Design review of the part built by this model. Coordinates are the model's own, in mm. A direction names the side the tool comes from. Round coordinates to 2 decimals unless told otherwise and drop trailing zeros. Loops run counter-clockwise (first coordinate to the right, second up) from the corner with the lowest first, then second, coordinate; pieces in that order, holes last. Notation, with made-up numbers: M -22,72.25 L 24,72.25 A29 ccw 24,105.25 Z; hole C 87,81 d6. An arc over 180 degrees is marked long. Answer as CSV lines item,"result". Start each with the question number.
Autodesk Inventor part; units mm, degrees
ref_plane "YZ Plane" through (0, 0, 0) normal (1, 0, 0) x (0, 1, 0)
ref_plane "XZ Plane" through (0, 0, 0) normal (0, 1, 0) x (-1, 0, 0)
ref_plane "XY Plane" through (0, 0, 0) normal (0, 0, 1) x (1, 0, 0)
sketch "Sketch1" plane through (0, 0, 0) normal (0, 1, 0) x (-1, 0, 0)
  line L0 (45.72, 0) -> (45.72, -69.85)
  line L1 (0, -69.85) -> (0, 0)
  line L2 (45.72, -69.85) -> (58.42, -69.85)
  line L3 (58.42, -69.85) -> (58.42, -82.55)
  line L4 (58.42, -82.55) -> (45.72, -82.55)
  line L5 (45.72, -82.55) -> (45.72, -69.85)
  line L6 (45.72, 0) -> (58.42, 0)
  line L7 (58.42, 0) -> (58.42, 12.7)
  line L8 (58.42, 12.7) -> (45.72, 12.7)
  line L9 (45.72, 12.7) -> (45.72, 0)
  line L10 (0, 0) -> (-12.7, 0)
  line L11 (-12.7, 0) -> (-12.7, 12.7)
  line L12 (-12.7, 12.7) -> (0, 12.7)
  line L13 (0, 12.7) -> (0, 0)
  line L14 (0, -69.85) -> (-12.7, -69.85)
  line L15 (-12.7, -69.85) -> (-12.7, -82.55)
  line L16 (-12.7, -82.55) -> (0, -82.55)
  line L17 (0, -82.55) -> (0, -69.85)
  line L18 (0, 0) -> (0, 6.35)
  line L19 (0, 6.35) -> (45.72, 6.35)
  line L20 (45.72, 6.35) -> (45.72, 0)
  line L21 (0, -69.85) -> (0, -76.2)
  line L22 (0, -76.2) -> (45.72, -76.2)
  line L23 (45.72, -76.2) -> (45.72, -69.85)
  line L24 (45.72, -69.85) -> (52.07, -69.85)
  line L25 (52.07, -69.85) -> (52.07, 0)
  line L26 (52.07, 0) -> (45.72, 0)
  line L27 (45.72, 0) -> (45.72, -69.85)
  line L28 (0, 0) -> (-8.636, 0)
  line L29 (-8.636, 0) -> (-8.636, -69.85)
  line L30 (-8.636, -69.85) -> (0, -69.85)
  line L31 (0, -69.85) -> (0, 0)
  line L32 (0, 3.175) -> (0, -9.525)
  line L33 (45.72, -9.525) -> (45.72, 3.175)
  line L34 (0, -73.025) -> (0, -60.325)
  line L35 (45.72, -60.325) -> (45.72, -73.025)
  line L36 (34.29, -60.325) -> (11.43, -60.325)
  line L37 (11.43, -60.325) -> (11.43, -73.025)
  line L38 (11.43, -73.025) -> (34.29, -73.025)
  line L39 (34.29, -73.025) -> (34.29, -60.325)
  line L40 (34.29, -9.525) -> (11.43, -9.525)
  line L41 (11.43, -9.525) -> (11.43, 3.175)
  line L42 (11.43, 3.175) -> (34.29, 3.175)
  line L43 (34.29, 3.175) -> (34.29, -9.525)
  line L44 (11.43, -3.175) -> (7.62, -3.175)
  line L45 (7.62, -3.175) -> (7.62, -6.985)
  line L46 (7.62, -6.985) -> (11.43, -6.985)
  line L47 (11.43, -6.985) -> (11.43, -3.175)
  line L48 (0, -6.985) -> (3.81, -6.985)
  line L49 (3.81, -6.985) -> (3.81, -10.795)
  line L50 (3.81, -10.795) -> (0, -10.795)
  line L51 (0, -10.795) -> (0, -6.985)
  line L52 (38.1, -62.865) -> (34.29, -62.865)
  line L53 (38.1, -66.675) -> (38.1, -62.865)
  line L54 (34.29, -66.675) -> (38.1, -66.675)
  line L55 (45.72, -62.865) -> (41.91, -62.865)
  line L56 (41.91, -62.865) -> (41.91, -59.055)
  line L57 (41.91, -59.055) -> (45.72, -59.055)
  line L58 (7.62, -62.865) -> (11.43, -62.865)
  line L59 (7.62, -66.675) -> (7.62, -62.865)
  line L60 (11.43, -66.675) -> (7.62, -66.675)
  line L61 (0, -62.865) -> (3.81, -62.865)
  line L62 (3.81, -62.865) -> (3.81, -59.055)
  line L63 (3.81, -59.055) -> (0, -59.055)
  line L64 (41.91, -10.795) -> (45.72, -10.795)
  line L65 (41.91, -6.985) -> (41.91, -10.795)
  line L66 (45.72, -6.985) -> (41.91, -6.985)
  line L67 (38.1, -6.985) -> (34.29, -6.985)
  line L68 (38.1, -3.175) -> (38.1, -6.985)
  line L69 (34.29, -3.175) -> (38.1, -3.175)
  line L70 (36.195, -10.795) -> (9.525, -10.795)
  line L71 (9.525, -10.795) -> (9.525, -59.055)
  line L72 (9.525, -59.055) -> (36.195, -59.055)
  line L73 (36.195, -59.055) -> (36.195, -10.795)
  line L74 (47.3075, -10.795) -> (50.4825, -10.795)
  line L75 (50.4825, -10.795) -> (50.4825, -59.055)
  line L76 (50.4825, -59.055) -> (47.3075, -59.055)
  line L77 (47.3075, -59.055) -> (47.3075, -10.795)
  line L78 (22.86, -34.925) -> (22.86, -41.845)
  line L79 (-1.5875, -10.795) -> (-4.7625, -10.795)
  line L80 (-4.7625, -10.795) -> (-4.7625, -59.055)
  line L81 (-4.7625, -59.055) -> (-1.5875, -59.055)
  line L82 (-1.5875, -59.055) -> (-1.5875, -10.795)
  dimension "d0" = 45.72
  dimension "d1" = 69.85
  dimension "d2" = 12.7
  dimension "d3" = 12.7
  dimension "d4" = 12.7
  dimension "d5" = 12.7
  dimension "d6" = 12.7
  dimension "d7" = 12.7
  dimension "d8" = 12.7
  dimension "d9" = 12.7
  dimension "d10" = 6.35
  dimension "d11" = 6.35
  dimension "d12" = 6.35
  dimension "d13" = 12.7
  dimension "d14" = 12.7
  dimension "d15" = 11.43
  dimension "d16" = 22.86
  dimension "d17" = 12.7
  dimension "d18" = 3.81
  dimension "d19" = 3.81
  dimension "d20" = 3.81
  dimension "d21" = 3.81
  dimension "d24" = 360
  dimension "d28" = 360
  dimension "d34" = 1.5875
  dimension "d35" = 3.175
extrude "Extrusion1" add sketch "Sketch1" along normal blind 2.54 contours L6 L25 L2 L0 | L9 L8 L7 L6 | L0 L66 L65 L64 L57 L56 L55 L5 L22 L17 L1 L61 L62 L63 L50 L49 L48 L13 L19 L9 | L2 L3 L4 L5 | L13 L10 L11 L12 | L1 L14 L29 L10 | L17 L16 L15 L14 | L73 L72 L71 L70
extrude "Extrusion2" add sketch "Sketch1" along normal blind 12.7 contours L0 L64 L65 L66 | L0 L55 L56 L57 | L48 L49 L50 L1 | L1 L63 L62 L61 | L52 L53 L54 L39 | L37 L60 L59 L58 | L43 L69 L68 L67 | L46 L45 L44 L41
fillet "Fillet1" radius 6.35 4 edges at (-58.42, 1.27, 12.7) (12.7, 1.27, 12.7) (12.7, 1.27, -82.55) (-58.42, 1.27, -82.55)
equation "\"BendRadius\" = Thickness"
equation "\"BendReliefWidth\" = Thickness"
equation "\"BendReliefDepth\" = 0.5 * Thickness"
equation "\"CornerReliefSize\" = 4 * Thickness"
equation "\"MinimumRemnant\" = 2 * Thickness"
equation "\"TransitionRadius\" = BendRadius"
equation "\"JacobiRadiusSize\" = BendRadius"
equation "\"GapSize\" = Thickness"
properties part number "PixfalconCover"
Item 1: Consider section A-A, the plane z = -71. Write out the cut boundary in (x, y), then the cut area to 3 significant figures.
Item 2: The part is to be moulded in two halves that separate along X. For faces 1 (the face through (-2, 8, -62.865)), 2 (the face through (-45.72, 8, -9)), 3 (the face through (-23, 1, -9.525)), say which applies: +X half, -X half, draft (parallel to the pull), parting line (faces both ways), or undercut.
Item 3: Consider section D-D, the plane x = -49. Write out the cut boundary in (y, z) (3 decimals).
Item 4: Tool access review of faces 4 (the face through (-10, 8, -3.175)), 5 (the face through (0, 8, -61)), 6 (the face through (-45.72, 1, 10)): name each direction out of +Z, -Z, +X, -X, +Y, -Y from which nothing blocks a thin tool from reaching the whole face with its end or side.
Item 5: Insertion check: pin 1 Ø5 at (x, y) = (-41.5, 6) entering from -Z (3 decimals); pin 2 Ø4 at (x, y) = (-10.5, 7) entering from +Z (3 decimals); pin 3 Ø1.9 at (y, z) = (6, -8.5) entering from -X; pin 4 Ø3 at (x, z) = (-42, -64) entering from +Y. Each pin has a flat end and moves straight along its axis. Give the tip position at first contact, or say it passes through.
Item 6: Consider section B-B, the plane y = 4.25. Count the separate pieces of the cut face and the enclosed holes in it, then the cut area to 3 significant figures.
Item 7: To check wall thickness, follow line 1 (Z direction, x = -14.5, y = 1.75) (3 decimals); line 2 (Z direction, x = -10, y = 2.75) (3 decimals); line 3 (X direction, y = 0.75, z = -51). State the ranges of each line that lie inside material, in increasing order.
Item 8: Consider section C-C, the plane z = -57.5. Write out the cut boundary in (x, y).
Found:
1,outline,"M -58.42,0 L -34.29,0 L -34.29,2.54 L -58.42,2.54 Z; M -11.43,0 L 12.7,0 L 12.7,2.54 L -11.43,2.54 Z"
1,area,"123 mm^2"
2,face 1,"draft"
2,face 2,"-X half"
2,face 3,"undercut"
3,outline,"M 0,-82.55 L 2.54,-82.55 L 2.54,-59.055 L 0,-59.055 Z; M 0,-10.795 L 2.54,-10.795 L 2.54,12.7 L 0,12.7 Z"
4,face 4,"+Z, +X, -X, +Y"
4,face 5,"+Z, -Z, +X, +Y"
4,face 6,"+Z, +Y, -Y"
5,pin 1,"stops at z = -62.865"
5,pin 2,"stops at z = -3.175"
5,pin 3,"stops at x = -45.72"
5,pin 4,"stops at y = 12.7"
6,separate pieces,"8"
6,enclosed holes,"0"
6,area,"116 mm^2"
7,line 1,"z = -76.2 to -73.025, -60.325 to -9.525, 3.175 to 6.35"
7,line 2,"z = -66.675 to -62.865, -6.985 to -3.175"
7,line 3,"x = -52.07 to -50.48, -47.31 to 1.59, 4.76 to 8.64"
8,outline,"M -52.07,0 L -50.48,0 L -50.48,2.54 L -52.07,2.54 Z; M -47.31,0 L 1.59,0 L 1.59,2.54 L -47.31,2.54 Z; M 4.76,0 L 8.64,0 L 8.64,2.54 L 4.76,2.54 Z"
